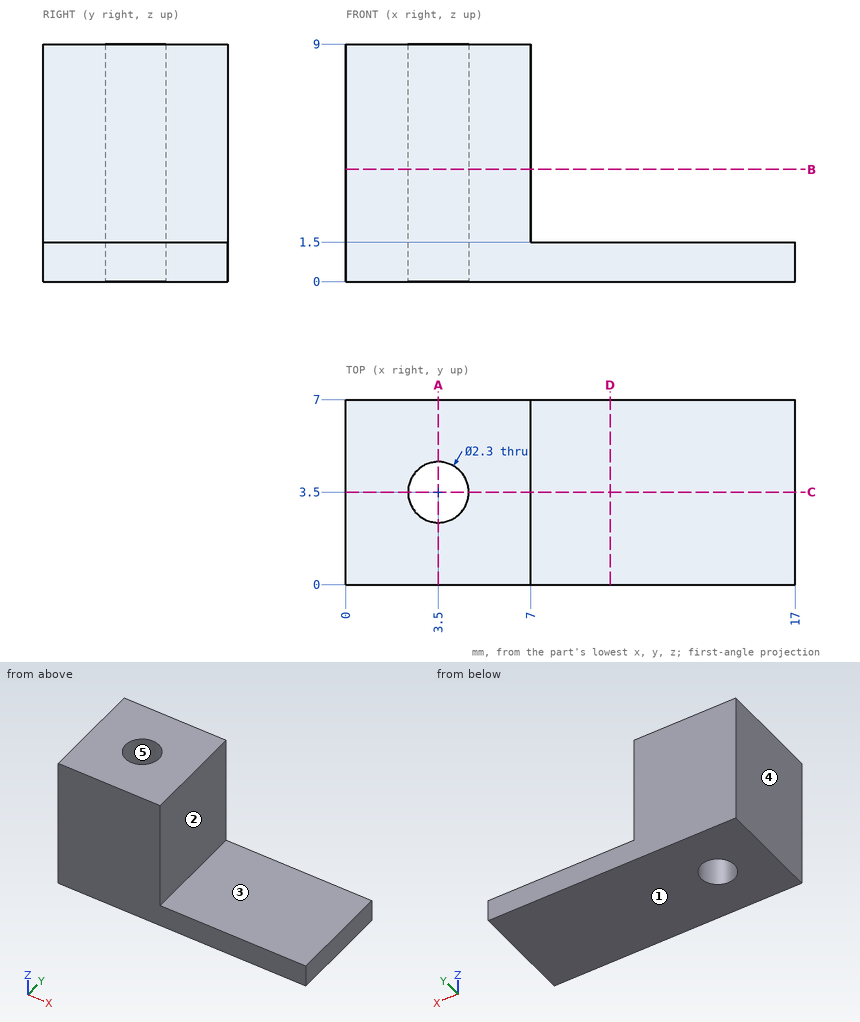
Geometry: see drawing. Coordinates: mm, zero at the bounding-box minimum. A direction names the side the tool comes from. Coordinates: 2 decimals unless noted, no trailing zeros. Order: outer loops, then holes, each group sorted by start corner. A loop starts at its lowest first (then second) coordinate and runs counter-clockwise, first axis right, second up. Notation, with made-up numbers: (-24.75, -25) - (-13.75, -25) arc R16 cw to (-13.75, -3) - close; hole circle Ø6 at (64, -35.75). An arc over 180 degrees is marked (long way). Write each question's results on one line, items separated by ' | '.
1) Pin query (flat end, axial travel): pin 1 (3 mm diameter, centred on x = 12.5, y = 1, fed in from +Z). Return the tip coordinate at first contact, or that it passes through.
Results list:
pin 1: z = 1.5
2) Set-up query: the marked faces 1 and 2. Return all of +Z, -Z, +X, -X, +Y, -Y with unobstructed straight access to the full face (end or side cutting, diameter ignored); none if empty.
Results list:
face 1: -Z, +X, -X, +Y, -Y | face 2: +Z, +X, +Y, -Y
3) Section B-B, the plane z = 4.25. Return loops of the section in (x, y), plus the area to 3 significant figures.
Results list:
outline: (0, 0) - (7, 0) - (7, 7) - (0, 7) - close; hole circle Ø2.3 at (3.5, 3.5) | area: 44.8 mm^2
4) Line query: line 1 (Y direction, x = 3.5, z = 5.5); line 2 (Z direction, x = 10.75, y = 1); line 3 (X direction, y = 3.25, z = 6.5). Output: solid intervals per line, ascending. Write a range as from..to.
Results list:
line 1: 0..2.35, 4.65..7 | line 2: 0..1.5 | line 3: 0..2.38, 4.62..7
5) Section D-D, the plane x = 10. Return loops of the section in (y, z), plus the area to 3 significant figures.
Results list:
outline: (0, 0) - (7, 0) - (7, 1.5) - (0, 1.5) - close | area: 10.5 mm^2
6) Section C-C, the plane y = 3.5. Return loops of the section in (x, z).
Results list:
outline: (0, 0) - (2.35, 0) - (2.35, 9) - (0, 9) - close; (4.65, 0) - (17, 0) - (17, 1.5) - (7, 1.5) - (7, 9) - (4.65, 9) - close
7) Section A-A, the plane x = 3.5. Return loops of the section in (y, z), plus the area to 3 significant figures.
Results list:
outline: (0, 0) - (2.35, 0) - (2.35, 9) - (0, 9) - close; (4.65, 0) - (7, 0) - (7, 9) - (4.65, 9) - close | area: 42.3 mm^2
8) Pull-direction query (X, two-part tool) for the marked faces 3, 4 and 5; classes: pulls with the +X half, pulls with the -X half, needs draft (parallel to the pull), parting line crosses it, or undercut.
Results list:
face 3: needs draft | face 4: pulls with the -X half | face 5: undercut
